from build123d import *

# Parameters (mm, degrees)
F0_W     = 60
F0_H     = 60
F1_DEPTH = 441
F3_D     = 16


with BuildPart() as f1:
    # F0 (on Front) → F1 (new body)
    with BuildSketch(Plane.XZ):
        Rectangle(F0_W, F0_H)
    extrude(amount=F1_DEPTH)

    # F3 (through all)
    with Locations(Plane.XY.offset(30)):
        with Locations((-15, -15), (15, -15), (-15, -35), (15, -35)):
            Hole(F3_D / 2)


solid = f1.part
Here's how the part is built. I have some questions about the finished solid (model axes, mm). Give positions to 0.01 mm unless a question says otherwise; leave off trailing zeros. Order: outer loops, then holes, each group sorted by start corner. A loop starts at its lowest first (then second) coordinate and runs counter-clockwise, first axis right, second up. Notation, with made-up numbers: M -22,-25.5 L 29,-25.5 A23 ccw 29,-17.5 Z; hole C 68,48 d3. An arc over 180 degrees is marked long. Answer as a JSON object with one key per item and string values. Group by question number.
1) Suppose I cut it at A-A, the plane x = 15. Write out the boundary of the cut face in (y, z).
2) I'm going to push flat-ended pins straight in: pin 1 Ø9.5 at (x, y) = (15, -15) entering from +Z; pin 2 Ø18.5 at (x, y) = (15, -35) entering from -Z. Where does each tip first touch, or does it pass through?
3) Suppose I cut it at C-C, the plane z = -18.5. Write out the boundary of the cut face in (x, y), plus the area to 3 significant figures.
4) Please list where these lines run through material, in increasing order: L1, parallel to Y at x = 15.5, z = 8; L2, parallel to X at y = -35.5, z = 18; L3, parallel to Y at x = 9.5, z = -12. Write a range as [from, to].
5) We'd pull the mould along X, two halves only. Please class faces 1 (the flat face through (30, -217, 0)), 2 (the flat face through (0, -217, 30)), 3 (the cylindrical face through (20.9, -29.6, -0.4)): pulls with the +X half, pulls with the -X half, needs draft (parallel to the pull), parting line crosses it, or undercut.
6) Suppose I cut it at B-B, the plane y = -15. Write out the boundary of the cut face in (x, z), plus the area to 3 significant figures.
Results found:
{
 "1": {"outline": "M -441,-30 L -43,-30 L -43,30 L -441,30 Z; M -27,-30 L -23,-30 L -23,30 L -27,30 Z; M -7,-30 L 0,-30 L 0,30 L -7,30 Z"},
 "2": {"pin 1": "through", "pin 2": "z = -30"},
 "3": {"outline": "M -30,-441 L 30,-441 L 30,0 L -30,0 Z; hole C -15,-35 d16; hole C -15,-15 d16; hole C 15,-35 d16; hole C 15,-15 d16", "area": "25,700 mm²"},
 "4": {"L1": "[-441, -42.98], [-27.02, -22.98], [-7.02, 0]", "L2": "[-30, -22.98], [-7.02, 7.02], [22.98, 30]", "L3": "[-441, -40.81], [-29.19, -20.81], [-9.19, 0]"},
 "5": {"face 1": "pulls with the +X half", "face 2": "needs draft", "face 3": "undercut"},
 "6": {"outline": "M -30,-30 L -23,-30 L -23,30 L -30,30 Z; M -7,-30 L 7,-30 L 7,30 L -7,30 Z; M 23,-30 L 30,-30 L 30,30 L 23,30 Z", "area": "1,680 mm²"}
}
